Source: three-view drawing plus pictorial views. Frame: mm from the lowest corner of the part. A direction names the side the tool comes from. Coordinates: 2 decimals unless noted, no trailing zeros. Order: outer loops, then holes, each group sorted by start corner. A loop starts at its lowest first (then second) coordinate and runs counter-clockwise, first axis right, second up. Notation, with made-up numbers: (-4.75, -37.75) -> (19.25, -37.75) arc R33 ccw to (19.25, -4.75) -> close; hole circle Ø1 at (-14.5, 39.5). An arc over 180 degrees is marked (long way). One line per question, with ' | ' between items.
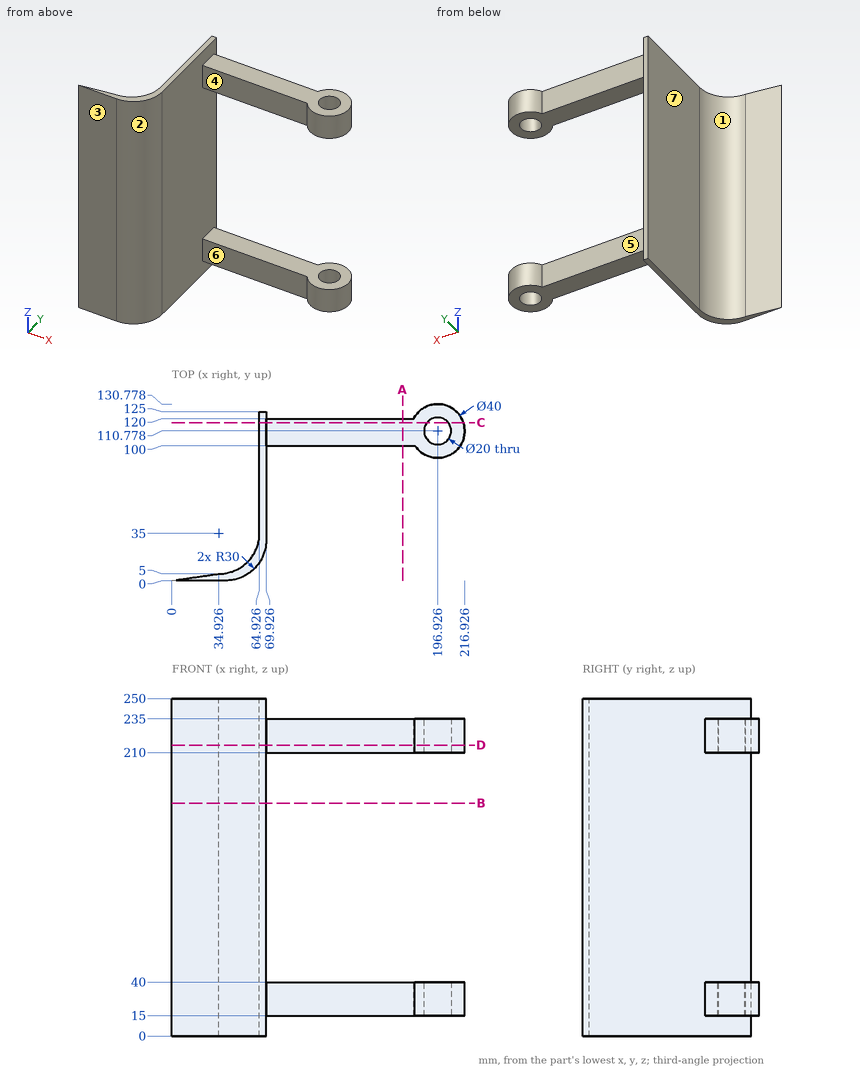
1. Cut plane C-C, the plane y = 117. Return loops of the section in (x, z).
Recorded:
outline: (64.93, 0) -> (69.93, 0) -> (69.93, 15) -> (189.1, 15) -> (189.1, 40) -> (69.93, 40) -> (69.93, 210) -> (189.1, 210) -> (189.1, 235) -> (69.93, 235) -> (69.93, 250) -> (64.93, 250) -> close; (204.75, 15) -> (215.93, 15) -> (215.93, 40) -> (204.75, 40) -> close; (204.75, 210) -> (215.93, 210) -> (215.93, 235) -> (204.75, 235) -> close
2. Cut plane A-A, the plane x = 171. Return loops of the section in (y, z).
Recorded:
outline: (100, 15) -> (120, 15) -> (120, 40) -> (100, 40) -> close; (100, 210) -> (120, 210) -> (120, 235) -> (100, 235) -> close
3. Cut plane B-B, the plane z = 172.5. Return loops of the section in (x, y), and give its area (3 significant figures).
Recorded:
outline: (0, 0) -> (39.93, 0) arc R30 ccw to (69.93, 30) -> (69.93, 125) -> (64.93, 125) -> (64.93, 35) arc R30 cw to (34.93, 5) -> close | area: 862 mm^2
4. Ray query, line 1 (Z direction, x = 123, y = 103.5); line 2 (X direction, y = 113, z = 163.5); line 3 (X direction, y = 113.5, z = 18). Return the intervals inside material, ascending. Write a range as [from, to].
Recorded:
line 1: z = [15, 40], [210, 235] | line 2: x = [64.93, 69.93] | line 3: x = [64.93, 187.3], [206.55, 216.74]
5. Cut plane D-D, the plane z = 215.5. Return loops of the section in (x, y), and give its area (3 significant figures).
Recorded:
outline: (0, 0) -> (39.93, 0) arc R30 ccw to (69.93, 30) -> (69.93, 100) -> (180.08, 100) arc R20 ccw (long way) to (179.18, 120) -> (69.93, 120) -> (69.93, 125) -> (64.93, 125) -> (64.93, 35) arc R30 cw to (34.93, 5) -> close; hole circle Ø20 at (196.93, 110.78) | area: 3,960 mm^2
6. Pin query (flat end, axial travel): pin 1 Ø12 at (x, y) = (137, 114.5) entering from +Z; pin 2 Ø4 at (y, z) = (79.5, 214) entering from -X; pin 3 Ø20 at (x, y) = (139.5, 111.5) entering from -Z. Return the tip coordinate at first contact, or that it passes through.
Recorded:
pin 1: stops at z = 235 | pin 2: stops at x = 64.93 | pin 3: stops at z = 15
7. Mould query, pull axis X, two halves, no side actions, for the marked faces 1, 2, 3 and 4. Classes: released by +X, released by -X, zero draft, split by the parting line, or undercut.
Recorded:
face 1: released by -X | face 2: released by +X | face 3: zero draft | face 4: undercut
8. Access query for the marked faces 5, 6 and 7. Directions: +Z, -Z, +X, -X, +Y, -Y. A direction counts if a zero-diameter tool reaches every point of the face in a straight line with its end or side. Return the directions, or none.
Recorded:
face 5: +Z, -Z, +Y | face 6: +Z, -Z, -Y | face 7: +Z, -Z, -X, +Y
